from build123d import *

# Parameters (mm, degrees)
SKETCH1_R                = 50
BOSS_EXTRUDE1_DEPTH      = 3
SKETCH2_R                = 7
BOSS_EXTRUDE2_DEPTH      = 5
CUT_EXTRUDE1_DEPTH       = 5
SKETCH4_R                = 2
CUT_EXTRUDE2_DEPTH       = 1.5
FILLET1_R                = 2
CIRPATTERN4_COUNT        = 16
FILLET1_OF_CIRPATTERN4_R = 2


with BuildPart() as part:
    # Sketch1 → Boss-Extrude1 (new body)
    with BuildSketch(Plane.XY):
        Circle(SKETCH1_R)
    extrude(amount=-BOSS_EXTRUDE1_DEPTH)

    # Sketch2 → Boss-Extrude2 (add)
    with BuildSketch(Plane.XY):
        Circle(SKETCH2_R)
    extrude(amount=BOSS_EXTRUDE2_DEPTH)

    # Sketch3 → Cut-Extrude1 (cut)
    with BuildSketch(Plane.XY.offset(5)):
        with BuildLine():
            Line((-1.625, 2.156240942), (-1.625, -2.156240942))
            ThreePointArc((-1.625, -2.156240942), (0, -2.7), (1.625, -2.156240942))
            Line((1.625, -2.156240942), (1.625, 2.156240942))
            ThreePointArc((1.625, 2.156240942), (0, 2.7), (-1.625, 2.156240942))
        make_face()
    extrude(amount=-CUT_EXTRUDE1_DEPTH, mode=Mode.SUBTRACT)

    # Sketch4 → Cut-Extrude2 (cut)
    with BuildSketch(Plane(origin=(0, 0, -3), x_dir=(-1, 0, 0), z_dir=(0, 0, -1))):
        with Locations((0, 44.850000011)):
            Circle(SKETCH4_R)
    cut_extrude2 = extrude(amount=-CUT_EXTRUDE2_DEPTH, mode=Mode.SUBTRACT)

    # Fillet1
    # the kernel refuses this fillet: 2 mm, written as the material it adds along each edge
    with BuildSketch(Plane(origin=(0, 44.850000011, -1.5), x_dir=(-1, 0, 0), z_dir=(0, -1, 0))) as fillet1_piece_1:
        with BuildLine():
            CenterArc((0.063508327, 2), FILLET1_R, 270, 75.522487814)
            Line((0.063508327, 0), (0.063508327, -0.04))
            Line((0.063508327, -0.04), (2, -0.04))
            Line((2, -0.04), (2.04, 0))
            ThreePointArc((2.04, 0), (2.04, 0.75), (2.038729833, 1.49))
            Line((2.038729833, 1.49), (2, 1.5))
        make_face()
    revolve(axis=Axis((0, 44.850000011, -1.5), (0, 0, -1)))

    # CirPattern4: Cut-Extrude2 ×16 about axis
    cirpattern4_axis = Axis((0, 0, 0), (0, 0, 1))
    for i in range(1, CIRPATTERN4_COUNT):
        add(cut_extrude2.rotate(cirpattern4_axis, i * 360 / CIRPATTERN4_COUNT), mode=Mode.SUBTRACT)

    # Fillet1 of CirPattern4
    # the kernel refuses this fillet: 2 mm, written as the material it adds along each edge
    with BuildSketch(Plane(origin=(-17.163351946, 41.435997043, -1.5), x_dir=(-0.9238795325112861, -0.3826834323650914, 0), z_dir=(0.3826834323650914, -0.9238795325112861, 0))) as fillet1_of_cirpattern4_piece_1:
        with BuildLine():
            CenterArc((0.063508327, 2), FILLET1_OF_CIRPATTERN4_R, 270, 75.522487814)
            Line((0.063508327, 0), (0.063508327, -0.04))
            Line((0.063508327, -0.04), (2, -0.04))
            Line((2, -0.04), (2.04, 0))
            ThreePointArc((2.04, 0), (2.04, 0.75), (2.038729833, 1.49))
            Line((2.038729833, 1.49), (2, 1.5))
        make_face()
    revolve(axis=Axis((-17.163351946, 41.435997043, -1.5), (0, 0, -1)))
    with BuildSketch(Plane(origin=(-31.713739144, 31.713739144, -1.5), x_dir=(-0.7071067811865467, -0.7071067811865485, 0), z_dir=(0.7071067811865485, -0.7071067811865467, 0))) as fillet1_of_cirpattern4_piece_2:
        with BuildLine():
            CenterArc((0.063508327, 2), FILLET1_OF_CIRPATTERN4_R, 270, 75.522487814)
            Line((0.063508327, 0), (0.063508327, -0.04))
            Line((0.063508327, -0.04), (2, -0.04))
            Line((2, -0.04), (2.04, 0))
            ThreePointArc((2.04, 0), (2.04, 0.75), (2.038729833, 1.49))
            Line((2.038729833, 1.49), (2, 1.5))
        make_face()
    revolve(axis=Axis((-31.713739144, 31.713739144, -1.5), (0, 0, -1)))
    with BuildSketch(Plane(origin=(-41.435997043, 17.163351946, -1.5), x_dir=(-0.3826834323650911, -0.9238795325112863, 0), z_dir=(0.9238795325112863, -0.3826834323650911, 0))) as fillet1_of_cirpattern4_piece_3:
        with BuildLine():
            CenterArc((0.063508327, 2), FILLET1_OF_CIRPATTERN4_R, 270, 75.522487814)
            Line((0.063508327, 0), (0.063508327, -0.04))
            Line((0.063508327, -0.04), (2, -0.04))
            Line((2, -0.04), (2.04, 0))
            ThreePointArc((2.04, 0), (2.04, 0.75), (2.038729833, 1.49))
            Line((2.038729833, 1.49), (2, 1.5))
        make_face()
    revolve(axis=Axis((-41.435997043, 17.163351946, -1.5), (0, 0, -1)))
    with BuildSketch(Plane(origin=(-44.850000011, 0, -1.5), x_dir=(0, -1, 0), z_dir=(1, 0, 0))) as fillet1_of_cirpattern4_piece_4:
        with BuildLine():
            CenterArc((0.063508327, 2), FILLET1_OF_CIRPATTERN4_R, 270, 75.522487814)
            Line((0.063508327, 0), (0.063508327, -0.04))
            Line((0.063508327, -0.04), (2, -0.04))
            Line((2, -0.04), (2.04, 0))
            ThreePointArc((2.04, 0), (2.04, 0.75), (2.038729833, 1.49))
            Line((2.038729833, 1.49), (2, 1.5))
        make_face()
    revolve(axis=Axis((-44.850000011, 0, -1.5), (0, 0, -1)))
    with BuildSketch(Plane(origin=(-41.435997043, -17.163351946, -1.5), x_dir=(0.3826834323650914, -0.9238795325112861, 0), z_dir=(0.9238795325112861, 0.3826834323650914, 0))) as fillet1_of_cirpattern4_piece_5:
        with BuildLine():
            CenterArc((0.063508327, 2), FILLET1_OF_CIRPATTERN4_R, 270, 75.522487814)
            Line((0.063508327, 0), (0.063508327, -0.04))
            Line((0.063508327, -0.04), (2, -0.04))
            Line((2, -0.04), (2.04, 0))
            ThreePointArc((2.04, 0), (2.04, 0.75), (2.038729833, 1.49))
            Line((2.038729833, 1.49), (2, 1.5))
        make_face()
    revolve(axis=Axis((-41.435997043, -17.163351946, -1.5), (0, 0, -1)))
    with BuildSketch(Plane(origin=(-31.713739144, -31.713739144, -1.5), x_dir=(0.7071067811865485, -0.7071067811865467, 0), z_dir=(0.7071067811865467, 0.7071067811865485, 0))) as fillet1_of_cirpattern4_piece_6:
        with BuildLine():
            CenterArc((0.063508327, 2), FILLET1_OF_CIRPATTERN4_R, 270, 75.522487814)
            Line((0.063508327, 0), (0.063508327, -0.04))
            Line((0.063508327, -0.04), (2, -0.04))
            Line((2, -0.04), (2.04, 0))
            ThreePointArc((2.04, 0), (2.04, 0.75), (2.038729833, 1.49))
            Line((2.038729833, 1.49), (2, 1.5))
        make_face()
    revolve(axis=Axis((-31.713739144, -31.713739144, -1.5), (0, 0, -1)))
    with BuildSketch(Plane(origin=(-17.163351946, -41.435997043, -1.5), x_dir=(0.9238795325112863, -0.3826834323650911, 0), z_dir=(0.3826834323650911, 0.9238795325112863, 0))) as fillet1_of_cirpattern4_piece_7:
        with BuildLine():
            CenterArc((0.063508327, 2), FILLET1_OF_CIRPATTERN4_R, 270, 75.522487814)
            Line((0.063508327, 0), (0.063508327, -0.04))
            Line((0.063508327, -0.04), (2, -0.04))
            Line((2, -0.04), (2.04, 0))
            ThreePointArc((2.04, 0), (2.04, 0.75), (2.038729833, 1.49))
            Line((2.038729833, 1.49), (2, 1.5))
        make_face()
    revolve(axis=Axis((-17.163351946, -41.435997043, -1.5), (0, 0, -1)))
    with BuildSketch(Plane(origin=(0, -44.850000011, -1.5), x_dir=(1, 0, 0), z_dir=(0, 1, 0))) as fillet1_of_cirpattern4_piece_8:
        with BuildLine():
            CenterArc((0.063508327, 2), FILLET1_OF_CIRPATTERN4_R, 270, 75.522487814)
            Line((0.063508327, 0), (0.063508327, -0.04))
            Line((0.063508327, -0.04), (2, -0.04))
            Line((2, -0.04), (2.04, 0))
            ThreePointArc((2.04, 0), (2.04, 0.75), (2.038729833, 1.49))
            Line((2.038729833, 1.49), (2, 1.5))
        make_face()
    revolve(axis=Axis((0, -44.850000011, -1.5), (0, 0, -1)))
    with BuildSketch(Plane(origin=(17.163351946, -41.435997043, -1.5), x_dir=(0.9238795325112864, 0.3826834323650908, 0), z_dir=(-0.3826834323650908, 0.9238795325112864, 0))) as fillet1_of_cirpattern4_piece_9:
        with BuildLine():
            CenterArc((0.063508327, 2), FILLET1_OF_CIRPATTERN4_R, 270, 75.522487814)
            Line((0.063508327, 0), (0.063508327, -0.04))
            Line((0.063508327, -0.04), (2, -0.04))
            Line((2, -0.04), (2.04, 0))
            ThreePointArc((2.04, 0), (2.04, 0.75), (2.038729833, 1.49))
            Line((2.038729833, 1.49), (2, 1.5))
        make_face()
    revolve(axis=Axis((17.163351946, -41.435997043, -1.5), (0, 0, -1)))
    with BuildSketch(Plane(origin=(31.713739144, -31.713739144, -1.5), x_dir=(0.7071067811865467, 0.7071067811865485, 0), z_dir=(-0.7071067811865485, 0.7071067811865467, 0))) as fillet1_of_cirpattern4_piece_10:
        with BuildLine():
            CenterArc((0.063508327, 2), FILLET1_OF_CIRPATTERN4_R, 270, 75.522487814)
            Line((0.063508327, 0), (0.063508327, -0.04))
            Line((0.063508327, -0.04), (2, -0.04))
            Line((2, -0.04), (2.04, 0))
            ThreePointArc((2.04, 0), (2.04, 0.75), (2.038729833, 1.49))
            Line((2.038729833, 1.49), (2, 1.5))
        make_face()
    revolve(axis=Axis((31.713739144, -31.713739144, -1.5), (0, 0, -1)))
    with BuildSketch(Plane(origin=(41.435997043, -17.163351946, -1.5), x_dir=(0.3826834323650908, 0.9238795325112864, 0), z_dir=(-0.9238795325112864, 0.3826834323650908, 0))) as fillet1_of_cirpattern4_piece_11:
        with BuildLine():
            CenterArc((0.063508327, 2), FILLET1_OF_CIRPATTERN4_R, 270, 75.522487814)
            Line((0.063508327, 0), (0.063508327, -0.04))
            Line((0.063508327, -0.04), (2, -0.04))
            Line((2, -0.04), (2.04, 0))
            ThreePointArc((2.04, 0), (2.04, 0.75), (2.038729833, 1.49))
            Line((2.038729833, 1.49), (2, 1.5))
        make_face()
    revolve(axis=Axis((41.435997043, -17.163351946, -1.5), (0, 0, -1)))
    with BuildSketch(Plane(origin=(44.850000011, 0, -1.5), x_dir=(0, 1, 0), z_dir=(-1, 0, 0))) as fillet1_of_cirpattern4_piece_12:
        with BuildLine():
            CenterArc((0.063508327, 2), FILLET1_OF_CIRPATTERN4_R, 270, 75.522487814)
            Line((0.063508327, 0), (0.063508327, -0.04))
            Line((0.063508327, -0.04), (2, -0.04))
            Line((2, -0.04), (2.04, 0))
            ThreePointArc((2.04, 0), (2.04, 0.75), (2.038729833, 1.49))
            Line((2.038729833, 1.49), (2, 1.5))
        make_face()
    revolve(axis=Axis((44.850000011, 0, -1.5), (0, 0, -1)))
    with BuildSketch(Plane(origin=(41.435997043, 17.163351946, -1.5), x_dir=(-0.3826834323650914, 0.9238795325112861, 0), z_dir=(-0.9238795325112861, -0.3826834323650914, 0))) as fillet1_of_cirpattern4_piece_13:
        with BuildLine():
            CenterArc((0.063508327, 2), FILLET1_OF_CIRPATTERN4_R, 270, 75.522487814)
            Line((0.063508327, 0), (0.063508327, -0.04))
            Line((0.063508327, -0.04), (2, -0.04))
            Line((2, -0.04), (2.04, 0))
            ThreePointArc((2.04, 0), (2.04, 0.75), (2.038729833, 1.49))
            Line((2.038729833, 1.49), (2, 1.5))
        make_face()
    revolve(axis=Axis((41.435997043, 17.163351946, -1.5), (0, 0, -1)))
    with BuildSketch(Plane(origin=(31.713739144, 31.713739144, -1.5), x_dir=(-0.7071067811865485, 0.7071067811865467, 0), z_dir=(-0.7071067811865467, -0.7071067811865485, 0))) as fillet1_of_cirpattern4_piece_14:
        with BuildLine():
            CenterArc((0.063508327, 2), FILLET1_OF_CIRPATTERN4_R, 270, 75.522487814)
            Line((0.063508327, 0), (0.063508327, -0.04))
            Line((0.063508327, -0.04), (2, -0.04))
            Line((2, -0.04), (2.04, 0))
            ThreePointArc((2.04, 0), (2.04, 0.75), (2.038729833, 1.49))
            Line((2.038729833, 1.49), (2, 1.5))
        make_face()
    revolve(axis=Axis((31.713739144, 31.713739144, -1.5), (0, 0, -1)))
    with BuildSketch(Plane(origin=(17.163351946, 41.435997043, -1.5), x_dir=(-0.9238795325112864, 0.3826834323650908, 0), z_dir=(-0.3826834323650908, -0.9238795325112864, 0))) as fillet1_of_cirpattern4_piece_15:
        with BuildLine():
            CenterArc((0.063508327, 2), FILLET1_OF_CIRPATTERN4_R, 270, 75.522487814)
            Line((0.063508327, 0), (0.063508327, -0.04))
            Line((0.063508327, -0.04), (2, -0.04))
            Line((2, -0.04), (2.04, 0))
            ThreePointArc((2.04, 0), (2.04, 0.75), (2.038729833, 1.49))
            Line((2.038729833, 1.49), (2, 1.5))
        make_face()
    revolve(axis=Axis((17.163351946, 41.435997043, -1.5), (0, 0, -1)))


solid = part.part
Build history of the part. All positions in model axes, mm. A direction names the side the tool comes from. Round coordinates to 2 decimals unless told otherwise and drop trailing zeros. Write each loop counter-clockwise with the first axis right and the second up, starting at its lowest first coordinate (ties: lowest second). Pieces come first, ordered by that corner, then holes. Notation, with made-up numbers: M 15.5,81.5 L 64.5,81.5 A22 cw 64.5,109.5 Z; hole C 58,-29.5 d1. An arc over 180 degrees is marked long. Answer as a JSON object with one key per item and string values. Group by question number.
(1) Cut at C-C (x = 11). Give the cut face in (y, z) (3 decimals).
(2) Which spindle directions (+Z, -Z, +X, -X, +Y, -Y) get a long thin tool onto all of the face, cutting with end or side? Do faces 1 (the flat face through (-2, 0, 5)), 2 (the flat face through (0, 0, 0)). Say none if no direction does.
(3) Cut at B-B (y = 5.5). Give the cut face in (x, z).
(4) Cut at A-A (z = 2). Give the cut face in (x, y) (3 decimals), and give its area (3 significant figures).
(5) Cut at D-D (x = -11.5). Give the cut face in (y, z).
(6) Flat gauge pins, fed straight in: pin 1 (2 mm diameter, centred on x = -40, z = 0.5, fed in from -Y); pin 2 (4 mm diameter, centred on x = -6, y = -37, fed in from +Z); pin 3 (3.5 mm diameter, centred on y = -1, z = 2.5, fed in from -X). Where does each tip first touch, or does it go through?
(7) Drill centre lines: L1, parallel to Z at x = 14, y = -2; L2, parallel to X at y = 1, z = 0.75 (3 decimals); L3, parallel to Y at x = 3, z = 1. Where is each one in solid material? Low to high.
(8) Mould opens along X. For faces 3 (the cylindrical face through (0, -2.7, 2.5)), 4 (the cylindrical face through (47.69, 15.02, -1.48)), 5 (the flat face through (-1, 1, -3)) say: pulls with the +X half, pulls with the -X half, needs draft (parallel to the pull), parting line crosses it, or undercut.
Responses:
{
 "1": {"outline": "M -48.775,-3 L 48.775,-3 L 48.775,0 L -48.775,0 Z"},
 "2": {"face 1": "+Z, +X, -X, +Y, -Y", "face 2": "+Z"},
 "3": {"outline": "M -49.7,-3 L 49.7,-3 L 49.7,0 L 4.33,0 L 4.33,5 L -4.33,5 L -4.33,0 L -49.7,0 Z"},
 "4": {"outline": "C 0,0 d14; hole M -1.625,-2.156 A2.7 ccw 1.625,-2.156 L 1.625,2.156 A2.7 ccw -1.625,2.156 Z", "area": "138 mm2"},
 "5": {"outline": "M -48.66,-3 L 48.66,-3 L 48.66,0 L -48.66,0 Z"},
 "6": {"pin 1": "stops at y = -31.12", "pin 2": "stops at z = 0", "pin 3": "stops at x = -7"},
 "7": {"L1": "z = -3 to 0", "L2": "x = -6.928 to -1.625, 1.625 to 6.928", "L3": "y = -6.32 to 6.32"},
 "8": {"face 3": "undercut", "face 4": "parting line crosses it", "face 5": "needs draft"}
}
